Source: CAD feature listing. Evaluate the final solid. Frame: model axes, mm. A direction names the side the tool comes from. Coordinates: 2 decimals unless noted, no trailing zeros. Write each loop counter-clockwise with the first axis right and the second up, starting at its lowest first coordinate (ties: lowest second). Pieces come first, ordered by that corner, then holes. Notation, with made-up numbers: (8, -26) -> (47, -26) arc R26 cw to (47, 6) -> close; hole circle Ø4 at (-23.5, 31). An arc over 180 degrees is marked (long way). Write item = value, one per line.
from build123d import *

# Parameters (mm, degrees)
SKETCH_1_W          = 39.9
SKETCH_1_H          = 20
SKETCH_1_R          = 1.5
EXTRUDE_1_DEPTH     = 4
EXTRUDE_4_DEPTH     = 20
SKETCH_7_R          = 1.5
CUT_EXTRUDE_3_DEPTH = 15
SKETCH_8_W          = 25
SKETCH_8_H          = 23
EXTRUDE_5_DEPTH     = 7.83
SKETCH_9_W          = 20
SKETCH_9_H          = 4
CUT_EXTRUDE_4_DEPTH = 20
FILLET_1_R          = 5
SKETCH_12_W         = 20
SKETCH_12_H         = 23
CUT_EXTRUDE_5_DEPTH = 2
SKETCH_14_W         = 20
SKETCH_14_H         = 5.83
EXTRUDE_6_DEPTH     = 3
CHAMFER_1_SIZE      = 1
CUT_EXTRUDE_6_DEPTH = 10


with BuildPart() as part:
    # 草图1 → 凸台-拉伸1 (new body)
    with BuildSketch(Plane(origin=(0, 0, 0), x_dir=(1, 0, 0), z_dir=(0, 1, 0))):
        Rectangle(SKETCH_1_W, SKETCH_1_H)
        with Locations(Location((8, 7.5, 0), (0, 0, 270))):
            Circle(SKETCH_1_R, mode=Mode.SUBTRACT)
        with Locations(Location((8, -7.5, 0), (0, 0, 90))):
            Circle(SKETCH_1_R, mode=Mode.SUBTRACT)
        with Locations(Location((-8, -7.5, 0), (0, 0, 270))):
            Circle(SKETCH_1_R, mode=Mode.SUBTRACT)
        with Locations(Location((-8, 7.5, 0), (0, 0, 90))):
            Circle(SKETCH_1_R, mode=Mode.SUBTRACT)
    extrude(amount=EXTRUDE_1_DEPTH)

    # 草图6 → 凸台-拉伸4 (add)
    with BuildSketch(Plane.ZY.offset(19.95)):
        Polygon((-10, 4), (10, 4), (17.83, 4), (17.83, -19), (10, -19), (10, 0), (-10, 0), align=None)
    extrude(amount=EXTRUDE_4_DEPTH)

    # 草图7 → 切除-拉伸3 (cut)
    with BuildSketch(Plane.XY.offset(17.83)):
        with Locations((-36, 2)):
            Circle(SKETCH_7_R)
        with Locations((-24, 2)):
            Circle(SKETCH_7_R)
        with Locations((-36, -15)):
            Circle(SKETCH_7_R)
        with Locations((-24, -15)):
            Circle(SKETCH_7_R)
    extrude(amount=-CUT_EXTRUDE_3_DEPTH, mode=Mode.SUBTRACT)

    # 草图8 → 凸台-拉伸5 (add)
    with BuildSketch(Plane.XY.offset(10)):
        with Locations((-7.45, -7.5)):
            Rectangle(SKETCH_8_W, SKETCH_8_H)
    extrude(amount=EXTRUDE_5_DEPTH)

    # 草图9 → 切除-拉伸4 (cut)
    with BuildSketch(Plane(origin=(0, 0, -10), x_dir=(-1, 0, 0), z_dir=(0, 0, -1))):
        with Locations((29.95, 2)):
            Rectangle(SKETCH_9_W, SKETCH_9_H)
    extrude(amount=-CUT_EXTRUDE_4_DEPTH, mode=Mode.SUBTRACT)

    # 圆角1
    fillet_1_edges = [part.edges().sort_by_distance(p)[0] for p in [
        (5.05, -7.5, 17.83),
    ]]
    fillet(fillet_1_edges, radius=FILLET_1_R)

    # 草图12 → 切除-拉伸5 (cut)
    with BuildSketch(Plane(origin=(0, 0, 10), x_dir=(-1, 0, 0), z_dir=(0, 0, -1))):
        with Locations((29.95, -7.5)):
            Rectangle(SKETCH_12_W, SKETCH_12_H)
    extrude(amount=-CUT_EXTRUDE_5_DEPTH, mode=Mode.SUBTRACT)

    # 草图14 → 凸台-拉伸6 (add)
    with BuildSketch(Plane(origin=(0, 4, 0), x_dir=(1, 0, 0), z_dir=(0, 1, 0))):
        with Locations((-29.95, -14.915)):
            Rectangle(SKETCH_14_W, SKETCH_14_H)
    extrude(amount=EXTRUDE_6_DEPTH)

    # 倒角1
    chamfer_1_edges = [part.edges().sort_by_distance(p)[0] for p in [
        (-19.95, -7.5, 12),
    ]]
    chamfer(chamfer_1_edges, length=CHAMFER_1_SIZE)

    # 草图16 → 切除-拉伸6 (cut)
    with BuildSketch(Plane.XY.offset(17.83)):
        Polygon((-19.95, 4), (-24.15, 4), (-25.95, 7), (-19.95, 7), align=None)
    extrude(amount=-CUT_EXTRUDE_6_DEPTH, mode=Mode.SUBTRACT)


solid = part.part
1) Cut plane B-B, the plane y = 2. Output: boundary loops of the cut face in (x, z), and give its area (3 significant figures).
Answer block:
outline = (-39.95, 12) -> (-37.5, 12) -> (-37.5, 17.83) -> (-39.95, 17.83) -> close; (-34.5, 12) -> (-25.5, 12) -> (-25.5, 17.83) -> (-34.5, 17.83) -> close; (-22.5, 12) -> (-20.95, 12) -> (-19.95, 11) -> (-19.95, -10) -> (19.95, -10) -> (19.95, 10) -> (5.05, 10) -> (5.05, 12.83) arc R5 ccw to (0.05, 17.83) -> (-22.5, 17.83) -> close; hole circle Ø3 at (-8, -7.5); hole circle Ø3 at (-8, 7.5); hole circle Ø3 at (8, -7.5); hole circle Ø3 at (8, 7.5)
area = 1,040 mm2
2) Material intervals for probe 1 along X at (y, z) = (1, 7.5); probe 2 along Y at (x, z) = (-24, 14.55); probe 3 along Y at (x, z) = (-36, 16.15), sorted ascending. Write a range as [from, to].
Answer block:
probe_1 = [-19.95, -9.5], [-6.5, 6.5], [9.5, 19.95]
probe_2 = [-19, -16.5], [-13.5, 0.5], [3.5, 4]
probe_3 = [-19, -16.5], [-13.5, 0.5], [3.5, 7]
3) Cut plane C-C, the plane z = -7.5. Output: boundary loops of the cut face in (x, y), and give its area (3 significant figures).
Answer block:
outline = (-19.95, 0) -> (-9.5, 0) -> (-9.5, 4) -> (-19.95, 4) -> close; (-6.5, 0) -> (6.5, 0) -> (6.5, 4) -> (-6.5, 4) -> close; (9.5, 0) -> (19.95, 0) -> (19.95, 4) -> (9.5, 4) -> close
area = 136 mm2
4) Cut plane A-A, the plane x = 8. Output: boundary loops of the cut face in (y, z).
Answer block:
outline = (0, -10) -> (4, -10) -> (4, -9) -> (0, -9) -> close; (0, -6) -> (4, -6) -> (4, 6) -> (0, 6) -> close; (0, 9) -> (4, 9) -> (4, 10) -> (0, 10) -> close
5) Pull-direction query (Y, two-part tool) for faces 6 (the flat face through (-18, -19, 14)), 7 (the cylindrical face through (-37.2, 1.1, 15)), 8 (the cylindrical face through (-7.1, 2, -6.3)); classes: +Y half, -Y half, draft (parallel to the pull), parting line (faces both ways), or undercut.
Answer block:
face_6 = -Y half
face_7 = undercut
face_8 = draft
6) Cut plane D-D, the plane z = 13.5. Output: boundary loops of the cut face in (x, y).
Answer block:
outline = (-39.95, -19) -> (5, -19) -> (5, 4) -> (-24.15, 4) -> (-25.95, 7) -> (-39.95, 7) -> close; hole circle Ø3 at (-36, -15); hole circle Ø3 at (-36, 2); hole circle Ø3 at (-24, -15); hole circle Ø3 at (-24, 2)
7) Reachability of faces 1 (the flat face through (-2, 4, 4)), 2 (the flat face through (0, 0, 0)), 3 (the flat face through (0, 2, -10)), 4 (the flat face through (12, 2, 10)), 5 (the flat face through (-19.95, 1, 1)) from +Z, -Z, +X, -X, +Y, -Y: full face, straight path, thin tool, end or side. Return the list, or none.
Answer block:
face_1 = +Z, -Z, +X, +Y
face_2 = -Z, +X, -X, -Y
face_3 = -Z, +X, -X, +Y, -Y
face_4 = +Z, +X, +Y, -Y
face_5 = -Z, -X, +Y, -Y
8) First-contact query: pin 1 Ø1.5 at (x, y) = (-31.5, -1) entering from -Z; pin 2 Ø3 at (x, y) = (15, 1) entering from +Z; pin 3 Ø8.5 at (x, z) = (-6.5, 2.5) entering from +Y; pin 4 Ø1.8 at (x, y) = (-24, -15) entering from +Z. Flat tips, straight axial feed; report the tip coordinate or a pass-through.
Answer block:
pin_1 = 12
pin_2 = 10
pin_3 = 4
pin_4 = through
